```python
from build123d import *

# Parameters (mm, degrees)
SKETCH1_W           = 35.2
SKETCH1_H           = 35.2
BOSS_EXTRUDE1_DEPTH = 34
SKETCH2_R           = 1.5
CUT_EXTRUDE1_DEPTH  = 4.5
SKETCH3_R           = 11
BOSS_EXTRUDE2_DEPTH = 2
SKETCH4_R           = 2.5
BOSS_EXTRUDE3_DEPTH = 22


with BuildPart() as part:
    # Sketch1 → Boss-Extrude1 (new body)
    with BuildSketch(Plane(origin=(0, 0, 0), x_dir=(1, 0, 0), z_dir=(0, 1, 0))):
        Rectangle(SKETCH1_W, SKETCH1_H)
    extrude(amount=BOSS_EXTRUDE1_DEPTH)

    # Sketch2 → Cut-Extrude1 (cut)
    with BuildSketch(Plane(origin=(0, 34, 0), x_dir=(1, 0, 0), z_dir=(0, 1, 0))):
        with Locations((-13, 13)):
            Circle(SKETCH2_R)
        with Locations((13, 13)):
            Circle(SKETCH2_R)
    cut_extrude1 = extrude(amount=-CUT_EXTRUDE1_DEPTH, mode=Mode.SUBTRACT)

    # Mirror1: Cut-Extrude1 across plane
    add(cut_extrude1.mirror(Plane.XY), mode=Mode.SUBTRACT)

    # Sketch3 → Boss-Extrude2 (add)
    with BuildSketch(Plane(origin=(0, 34, 0), x_dir=(1, 0, 0), z_dir=(0, 1, 0))):
        Circle(SKETCH3_R)
    extrude(amount=BOSS_EXTRUDE2_DEPTH)

    # Sketch4 → Boss-Extrude3 (add)
    with BuildSketch(Plane(origin=(0, 36, 0), x_dir=(1, 0, 0), z_dir=(0, 1, 0))):
        Circle(SKETCH4_R)
    extrude(amount=BOSS_EXTRUDE3_DEPTH)


solid = part.part
```
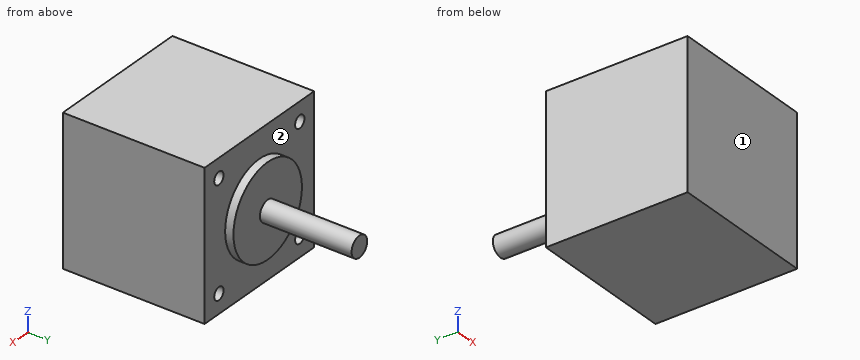
Model file for the job. Use its own axes, mm. Face numbers are marked on the shaded views. A direction names the side the tool comes from. Give positions to 0.01 mm unless a question says otherwise; leave off trailing zeros. Loops run counter-clockwise (first coordinate to the right, second up) from the corner with the lowest first, then second, coordinate; pieces in that order, holes last. Notation, with made-up numbers: (43, 71) - (58, 71) arc R20 ccw to (58, 84) - close; hole circle Ø2 at (-31.75, 54). An arc over 180 degrees is marked (long way). One line per item, written item: value. Start each with the question number.
1. Slice it at B-B (x = -13). List the corners of the cut face in (y, z), plus the area to 3 significant figures.
2. Slice it at D-D (z = 7.5). List the corners of the cut face in (x, y).
3. Pin check, flat tips, straight feed: pin 1 (6 mm diameter, centred on y = 39.5, z = -8, fed in from -X) (3 decimals); pin 2 (2.5 mm diameter, centred on x = 13, z = -12.5, fed in from +Y); pin 3 (12 mm diameter, centred on x = 3.5, z = 13.5, fed in from +Y); pin 4 (0.9 mm diameter, centred on x = -13.5, z = -13, fed in from +Y). Stop position of each tip, or through.
4. Slice it at C-C (x = 9.5). List the corners of the cut face in (y, z), plus the area to 3 significant figures.
5. Slice it at A-A (z = 0). List the corners of the cut face in (x, y), plus the area to 3 significant figures.
6. Which spindle directions (+Z, -Z, +X, -X, +Y, -Y) get a long thin tool onto all of the face, cutting with end or side? Do the marked faces 1 and 2. Say none if no direction does.
7. Probe L1, parallel to Z at x = -13, y = 31.4; L2, parallel to Y at x = -2, z = 10. List the from-to ranges inside material, lowest first. Write a range as from..to.
Solution:
1. outline: (0, -17.6) - (34, -17.6) - (34, -14.5) - (29.5, -14.5) - (29.5, -11.5) - (34, -11.5) - (34, 11.5) - (29.5, 11.5) - (29.5, 14.5) - (34, 14.5) - (34, 17.6) - (0, 17.6) - close
1. area: 1,170 mm^2
2. outline: (-17.6, 0) - (17.6, 0) - (17.6, 34) - (8.05, 34) - (8.05, 36) - (-8.05, 36) - (-8.05, 34) - (-17.6, 34) - close
3. pin 1: passes through
3. pin 2: stops at y = 34
3. pin 3: stops at y = 36
3. pin 4: stops at y = 29.5
4. outline: (0, -17.6) - (34, -17.6) - (34, -5.55) - (36, -5.55) - (36, 5.55) - (34, 5.55) - (34, 17.6) - (0, 17.6) - close
4. area: 1,220 mm^2
5. outline: (-17.6, 0) - (17.6, 0) - (17.6, 34) - (11, 34) - (11, 36) - (2.5, 36) - (2.5, 58) - (-2.5, 58) - (-2.5, 36) - (-11, 36) - (-11, 34) - (-17.6, 34) - close
5. area: 1,350 mm^2
6. face 1: +Z, -Z, +X, -X, -Y
6. face 2: +Y
7. L1: z = -17.6..-14.5, -11.5..11.5, 14.5..17.6
7. L2: y = 0..36
